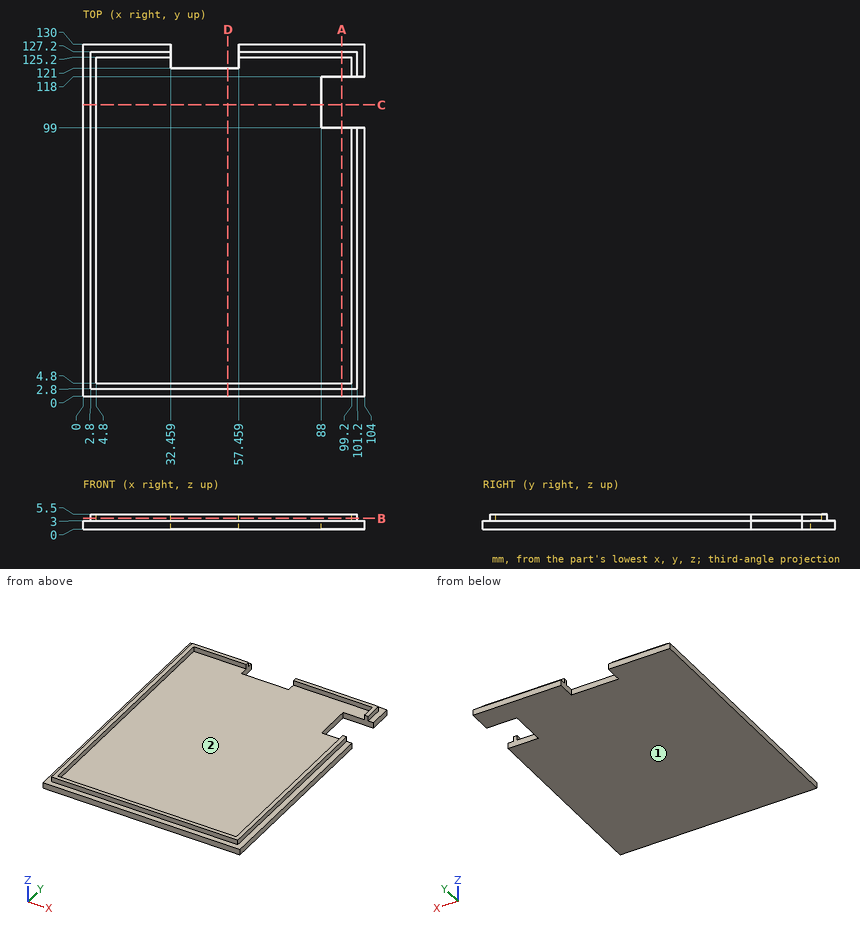
Answer from the drawing. Dimensions are ordinates in mm from the lowest x, y and z of the part. Give positions to 0.01 mm unless a question says otherwise; leave off trailing zeros. Order: outer loops, then holes, each group sorted by start corner. A loop starts at its lowest first (then second) coordinate and runs counter-clockwise, first axis right, second up. Notation, with made-up numbers: (-20.75, -30) -> (28.25, -30) arc R14 ccw to (28.25, -21) -> close; hole circle Ø3 at (65, 83). An arc over 180 degrees is marked (long way). Answer as a JSON object with one key per item and string values. Group by question number.
1. Flat-ended cylindrical pins translate along their axes: pin 1 Ø2 at (x, z) = (86.5, 4.5) entering from -Y; pin 2 Ø1.5 at (y, z) = (67, 4.5) entering from +X; pin 3 Ø1 at (x, y) = (66.5, 43) entering from +Z; pin 4 Ø5 at (x, y) = (48.5, 67) entering from -Z. Find the tip coordinate at first contact, or state that the pin passes through.
2. Section B-B on z = 3.95 is taken. Determine the outline of the cut face in (x, y).
3. Section A-A on x = 95.5 is taken. Determine the outline of the cut face in (y, z).
4. The mould has two halves that part along Y. Classify the marked faces 1 and 2: released by +Y, released by -Y, zero draft, split by the parting line, or undercut.
5. Section D-D on x = 53.5 is taken. Determine the outline of the cut face in (y, z), plus the area to 3 significant figures.
6. Section C-C on y = 107.5 is taken. Determine the outline of the cut face in (x, z).
7. Consider line 1 along Y through (x, z) = (18, 4.35); line 2 along Z through (x, y) = (96.5, 11); line 3 along X through (y, z) = (12, 3.9). Determine where each line is inside the solid, lowest interval first. Write a range as [from, to].
Result sheet:
{
 "1": {"pin 1": "stops at y = 2.8", "pin 2": "stops at x = 101.2", "pin 3": "stops at z = 3", "pin 4": "stops at z = 0"},
 "2": {"outline": "(2.8, 2.8) -> (101.2, 2.8) -> (101.2, 99) -> (99.2, 99) -> (99.2, 4.8) -> (4.8, 4.8) -> (4.8, 125.2) -> (32.46, 125.2) -> (32.46, 127.2) -> (2.8, 127.2) -> close; (57.46, 125.2) -> (99.2, 125.2) -> (99.2, 118) -> (101.2, 118) -> (101.2, 127.2) -> (57.46, 127.2) -> close"},
 "3": {"outline": "(0, 0) -> (99, 0) -> (99, 3) -> (4.8, 3) -> (4.8, 5.5) -> (2.8, 5.5) -> (2.8, 3) -> (0, 3) -> close; (118, 0) -> (130, 0) -> (130, 3) -> (127.2, 3) -> (127.2, 5.5) -> (125.2, 5.5) -> (125.2, 3) -> (118, 3) -> close"},
 "4": {"face 1": "zero draft", "face 2": "undercut"},
 "5": {"outline": "(0, 0) -> (121, 0) -> (121, 3) -> (4.8, 3) -> (4.8, 5.5) -> (2.8, 5.5) -> (2.8, 3) -> (0, 3) -> close", "area": "368 mm^2"},
 "6": {"outline": "(0, 0) -> (88, 0) -> (88, 3) -> (4.8, 3) -> (4.8, 5.5) -> (2.8, 5.5) -> (2.8, 3) -> (0, 3) -> close"},
 "7": {"line 1": "y = [2.8, 4.8], [125.2, 127.2]", "line 2": "z = [0, 3]", "line 3": "x = [2.8, 4.8], [99.2, 101.2]"}
}
